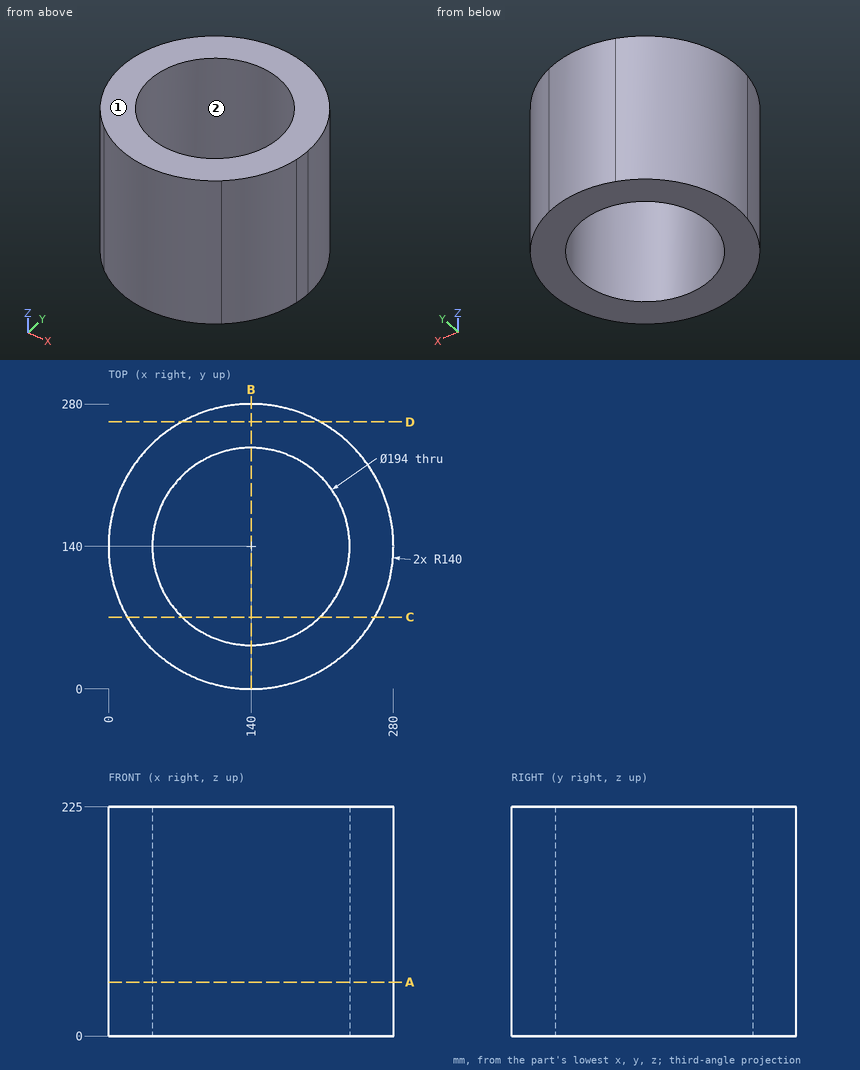
Input: dimensioned drawing with shaded views. Units: mm. Origin: part minimum x, y, z. Give positions to 0.01 mm unless a question says otherwise; leave off trailing zeros. Write each loop counter-clockwise with the first axis right and the second up, starting at its lowest first coordinate (ties: lowest second). Pieces come first, ordered by that corner, then holes. Notation, with made-up numbers: (-35, 77) -> (11, 77) arc R27 cw to (11, 106) -> close; hole circle Ø1 at (-1.75, 87). An arc over 180 degrees is marked (long way). Return JSON: item names as keys, results as strings. Group by question number.
1. Material intervals for line 1 (X direction, y = 128, z = 18) (1 decimal); line 2 (Y direction, x = 87, z = 22); line 3 (Y direction, x = 149.5, z = 65.5), sorted ascending. Write a range as from..to.
2. Section D-D, the plane y = 262.5. Output: boundary loops of the cut face in (x, z), then the cut area to 3 significant figures.
3. Section B-B, the plane x = 140. Output: boundary loops of the cut face in (y, z).
4. Mould query, pull axis Y, two halves, no side actions, for the marked faces 1 and 2. Classes: +Y half, -Y half, draft (parallel to the pull), parting line (faces both ways), or undercut.
5. Section C-C, the plane y = 70.5. Output: boundary loops of the cut face in (x, z), then the cut area to 3 significant figures.
6. Pin query (flat end, axial travel): pin 1 Ø5 at (x, z) = (117.5, 165.5) entering from -Y; pin 2 Ø1 at (y, z) = (29.5, 44.5) entering from +X; pin 3 Ø4 at (y, z) = (218.5, 79.5) entering from +X. Return the tip coordinate at first contact, or that it passes through.
7. Section A-A, the plane z = 53. Output: boundary loops of the cut face in (x, y) (1 decimal).
Determined:
{
 "1": {"line 1": "x = 0.5..43.7, 236.3..279.5", "line 2": "y = 10.42..58.76, 221.24..269.58", "line 3": "y = 0.32..43.47, 236.53..279.68"},
 "2": {"outline": "(72.22, 0) -> (207.78, 0) -> (207.78, 225) -> (72.22, 225) -> close", "area": "30,500 mm2"},
 "3": {"outline": "(0, 0) -> (43, 0) -> (43, 225) -> (0, 225) -> close; (237, 0) -> (280, 0) -> (280, 225) -> (237, 225) -> close"},
 "4": {"face 1": "draft", "face 2": "undercut"},
 "5": {"outline": "(18.47, 0) -> (72.33, 0) -> (72.33, 225) -> (18.47, 225) -> close; (207.67, 0) -> (261.53, 0) -> (261.53, 225) -> (207.67, 225) -> close", "area": "24,200 mm2"},
 "6": {"pin 1": "stops at y = 1.44", "pin 2": "stops at x = 226.6", "pin 3": "stops at x = 257.25"},
 "7": {"outline": "(51.8, 31.3) arc R140 ccw to (228.2, 31.3) arc R140 ccw to (278.2, 117.9) arc R140 ccw to (280, 140) arc R140 ccw to (190, 270.8) arc R140 ccw to (90, 270.8) arc R140 ccw to start; hole circle Ø194 at (140, 140)"}
}
